```python
from build123d import *

# Parameters (mm, degrees)
F0_W     = 12
F0_H     = 30
F0_R     = 3
F1_DEPTH = 5
F2_DEPTH = 10
F3_DEPTH = 5
F4_R     = 5.99999


# Not quite as in the source:
# - a fillet or chamfer is up to 0.001 mm smaller than in the source, because OpenCascade refuses the exact size


with BuildPart() as f1:
    # F0 (on Top) → F1 (new body)
    with BuildSketch(Plane.XY):
        with Locations((0.0119865412, -0.4361811298)):
            Rectangle(F0_W, F0_H)
        with Locations((0.0119865412, -9.4361811298)):
            Circle(F0_R, mode=Mode.SUBTRACT)
        with Locations((0.0119865412, 8.5638188702)):
            Circle(F0_R, mode=Mode.SUBTRACT)
        with Locations((0.0119865412, 8.5638188702)):
            Circle(F0_R)
        with Locations((0.0119865412, -9.4361811298)):
            Circle(F0_R)
    extrude(amount=F1_DEPTH)

    # F0 (on Top) → F2 (join)
    with BuildSketch(Plane.XY):
        with Locations((0.0119865412, 8.5638188702)):
            Circle(F0_R)
    extrude(amount=F2_DEPTH)

    # F0 (on Top) → F3 (join)
    with BuildSketch(Plane.XY):
        with Locations((0.0119865412, -9.4361811298)):
            Circle(F0_R)
    extrude(amount=-F3_DEPTH)

    # F4 (radius 6 in the source; OpenCascade refuses exactly that, so slightly less here)
    f4_edges = [f1.edges().sort_by_distance(p)[0] for p in [
        (6.011987, 14.563819, 2.5),
        (-5.988013, 14.563819, 2.5),
        (6.011987, -15.436181, 2.5),
        (-5.988013, -15.436181, 2.5),
    ]]
    fillet(f4_edges, radius=F4_R)


solid = f1.part
```
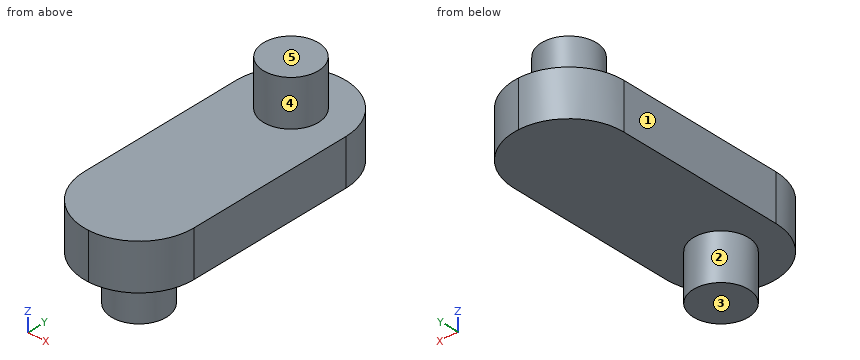
The listing builds one solid part. Answer for the finished solid, in the listing's coordinates (mm). Face numbers are marked on the shaded views. A direction names the side the tool comes from. Coordinates: 2 decimals unless noted, no trailing zeros. Write each loop counter-clockwise with the first axis right and the second up, starting at its lowest first coordinate (ties: lowest second). Pieces come first, ordered by that corner, then holes. Notation, with made-up numbers: (-37.75, -24) - (-30.75, -24) arc R24 ccw to (-30.75, -1) - close; hole circle Ø2 at (49, -1). An arc over 180 degrees is marked (long way). Return JSON: item names as keys, results as strings. Group by question number.
Q1. Which of the six approach directions +Z, -Z, +X, -X, +Y, -Y give full straight-line access (tool end or side, diameter ignored) to the marked faces 1 and 2?
Q2. Find the intervals of material crossed by line 1 along Z through (x, y) = (1.75, 4); line 2 along Y through (x, z) = (0.25, 3); line 3 along Z through (x, y) = (0.5, -9), in increasing order. Write a range as [from, to].
Q3. The part is cut by section B-B on x = 1.5. Write down the section's boundary in (y, z), and give its area (3 significant figures).
Q4. The part is cut by section D-D on z = -0.75. Write down the section's boundary in (x, y), and give its area (3 significant figures).
Q5. For a pull along Z with two mould halves and no side action, classify the marked faces 3, 4 and 5 as +Z half, -Z half, draft (parallel to the pull), parting line (faces both ways), or undercut.
Q6. Flat-ended cylindrical pins translate along their axes: pin 1 Ø1.5 at (x, y) = (-2.5, 4.5) entering from -Z; pin 2 Ø6 at (x, y) = (-3, -3.5) entering from +Z. Find the tip coordinate at first contact, or state that the pin passes through.
Q7. The part is cut by section C-C on y = 2.5. Write down the section's boundary in (x, z), and give its area (3 significant figures).
Evaluation:
{
 "1": {"face 1": "+Z, -Z, -X, +Y, -Y", "face 2": "-Z"},
 "2": {"line 1": "z = [0, 5]", "line 2": "y = [-15.43, 14.56]", "line 3": "z = [-5, 5]"},
 "3": {"outline": "(-15.25, 0) - (-12.04, 0) - (-12.04, -5) - (-6.83, -5) - (-6.83, 0) - (14.38, 0) - (14.38, 5) - (11.17, 5) - (11.17, 10) - (5.96, 10) - (5.96, 5) - (-15.25, 5) - close", "area": "200 mm2"},
 "4": {"outline": "circle Ø6 at (0.01, -9.44)", "area": "28.3 mm2"},
 "5": {"face 3": "-Z half", "face 4": "draft", "face 5": "+Z half"},
 "6": {"pin 1": "stops at z = 0", "pin 2": "stops at z = 5"},
 "7": {"outline": "(-5.99, 0) - (6.01, 0) - (6.01, 5) - (-5.99, 5) - close", "area": "60.0 mm2"}
}
